CAD build for the part. Positions are in the model's coordinates, mm. Face numbers are marked on the shaded views. A direction names the side the tool comes from. Give positions to 0.01 mm unless a question says otherwise; leave off trailing zeros. Write each loop counter-clockwise with the first axis right and the second up, starting at its lowest first coordinate (ties: lowest second). Pieces come first, ordered by that corner, then holes. Notation, with made-up numbers: (59, -11) - (71, -11) arc R29 cw to (71, 26) - close; hole circle Ø1 at (85, 31.25). An arc over 180 degrees is marked (long way). Answer as a JSON object with one key per item and string values.
from build123d import *

# Parameters (mm, degrees)
BOSS_EXTRUDE1_DEPTH = 42.8
SKETCH2_W           = 34.8
SKETCH2_H           = 38.311897311
CUT_EXTRUDE1_DEPTH  = 60.585181768
CHAMFER1_SIZE       = 2
FILLET1_R           = 1
CUT_EXTRUDE2_DEPTH  = 59.306444702


with BuildPart() as part:
    # Sketch1 → Boss-Extrude1 (new body)
    with BuildSketch(Plane(origin=(0, 0, 0), x_dir=(0, 0, -1), z_dir=(1, 0, 0))):
        with BuildLine():
            Line((-10, -6), (10, -6))
            Line((10, -6), (10, 6))
            ThreePointArc((10, 6), (9.25619767, 19.071476996), (7.034393072, 31.974202951))
            ThreePointArc((7.034393072, 31.974202951), (2.269388413, 36.269117533), (-3.402199146, 33.271676085))
            ThreePointArc((-3.402199146, 33.271676085), (-8.327095908, 20.029213205), (-10, 6))
            Line((-10, 6), (-10, -6))
        make_face()
        with BuildLine():
            ThreePointArc((0.001705571, 30.983312005), (-1.596543983, 17.513106187), (-1.778018244, 3.949628997))
            ThreePointArc((-1.778018244, 3.949628997), (-0.116879823, 2.413198345), (1.419550828, 4.074336766))
            ThreePointArc((1.419550828, 4.074336766), (1.596543983, 17.302893813), (3.15532829, 30.440482617))
            ThreePointArc((3.15532829, 30.440482617), (1.849931624, 32.288708671), (0.001705571, 30.983312005))
        make_face(mode=Mode.SUBTRACT)
    extrude(amount=BOSS_EXTRUDE1_DEPTH)

    # Sketch2 → Cut-Extrude1 (cut, through all)
    with BuildSketch(Plane.XY.offset(10)):
        with Locations((21.4, 17.155948656)):
            Rectangle(SKETCH2_W, SKETCH2_H)
    extrude(amount=-CUT_EXTRUDE1_DEPTH, mode=Mode.SUBTRACT)

    # Chamfer1
    chamfer1_edges = [part.edges().sort_by_distance(p)[0] for p in [
        (4, -2, 0),
        (38.8, -2, 0),
    ]]
    chamfer(chamfer1_edges, length=CHAMFER1_SIZE)

    # Fillet1
    fillet1_edges = [part.edges().sort_by_distance(p)[0] for p in [
        (42.8, 20.029213205, 8.327095908),
        (42.8, 0, 10),
        (42.8, -6, 0),
        (42.8, 0, -10),
        (0, 32.288708671, -1.849931624),
        (0, 17.513106187, 1.596543983),
        (0, 2.413198345, 0.116879823),
        (0, 17.302893813, -1.596543983),
        (42.8, 32.288708671, -1.849931624),
        (42.8, 17.513106187, 1.596543983),
        (42.8, 2.413198345, 0.116879823),
        (42.8, 17.302893813, -1.596543983),
        (42.8, 19.071476996, -9.25619767),
        (4, 36.269117533, -2.269388413),
        (4, 19.071476996, -9.25619767),
        (4, 3, -10),
        (4, 20.029213205, 8.327095908),
        (38.8, 19.071476996, -9.25619767),
        (38.8, 36.269117533, -2.269388413),
        (38.8, 20.029213205, 8.327095908),
        (4, 3, 10),
        (0, 0, -10),
        (0, -6, 0),
        (0, 0, 10),
        (42.8, 36.269117533, -2.269388413),
        (38.8, 3, -10),
        (38.8, 3, 10),
        (21.4, -2, 10),
        (0, 20.029213205, 8.327095908),
        (21.4, -2, -10),
        (6, -2, 0),
        (36.8, -2, 0),
        (37.8, -1, 10),
        (37.8, -1, -10),
        (5, -1, 10),
        (0, 36.269117533, -2.269388413),
        (5, -1, -10),
        (0, 19.071476996, -9.25619767),
    ]]
    fillet(fillet1_edges, radius=FILLET1_R)

    # Sketch3 → Cut-Extrude2 (cut, through all)
    with BuildSketch(Plane(origin=(0, -2, 0), x_dir=(1, 0, 0), z_dir=(0, 1, 0))):
        with BuildLine():
            Line((19.25, -2.5), (19.25, 2.5))
            ThreePointArc((19.25, 2.5), (21.4, 4.65), (23.55, 2.5))
            Line((23.55, 2.5), (23.55, -2.5))
            ThreePointArc((23.55, -2.5), (21.4, -4.65), (19.25, -2.5))
        make_face()
    extrude(amount=-CUT_EXTRUDE2_DEPTH, mode=Mode.SUBTRACT)


solid = part.part
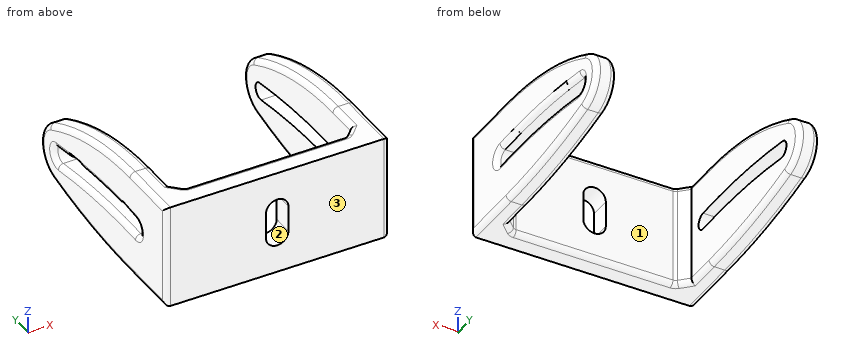
Item 1: Which spindle directions (+Z, -Z, +X, -X, +Y, -Y) get a long thin tool onto all of the face, cutting with end or side? Do the marked faces 1, 2 and 3. Say none if no direction does.
Entries:
{"face 1": "+Z, -Z, +Y", "face 2": "+Y, -Y", "face 3": "+Z, -Z, +X, -X, -Y"}
Item 2: Flat gauge pins, fed straight in: P1, Ø9, axis at x = 27, z = -2.5, coming from the +Y side; P2, Ø6, axis at y = 22.5, z = -1.5, coming from the -X side; P3, Ø1, axis at x = 37.5, z = -2.5, coming from the +Y side. Where does each tip first touch, or does it go through?
Entries:
{"P1": "y = -2", "P2": "x = 0", "P3": "y = -0.8"}
Item 3: Cut at B-B (y = 10.5). State how many separate pieces and enclosed holes the cut face has, and give its area (3 significant figures).
Entries:
{"separate pieces": "4", "enclosed holes": "0", "area": "130 mm2"}
Item 4: Cut at C-C (x = 15.5). Give the cut face in (y, z).
Entries:
{"outline": "(-6, -10) - (-3, -10) arc R1 ccw to (-2, -9) - (-2, 9) arc R1 ccw to (-3, 10) - (-6, 10) - close"}
Item 5: Cut at A-A (x = 21.4). Give the cut face in (y, z), and give its area (3 significant figures).
Entries:
{"outline": "(-6, -10) - (-3, -10) arc R1 ccw to (-2, -9) - (-2, -4.65) - (-6, -4.65) - close; (-6, 4.65) - (-2, 4.65) - (-2, 9) arc R1 ccw to (-3, 10) - (-6, 10) - close", "area": "42.4 mm2"}
Item 6: Probe line 1 (X direction, y = 1.5, z = -2.5); line 2 (Y direction, x = 30.5, z = 2); line 3 (Z direction, x = 39, y = 12.5). List the from-to ranges inside material, lowest first. Write a range as from..to.
Entries:
{"line 1": "0..4, 38.8..42.8", "line 2": "-6..-2", "line 3": "-9.42..-1.37, 1.83..9.24"}
